Job drawing, mm, ordinate dimensions from the low corner. One solid piece. A direction names the side the tool comes from. Round coordinates to 2 decimals unless told otherwise and drop trailing zeros. Order: outer loops, then holes, each group sorted by start corner. A loop starts at its lowest first (then second) coordinate and runs counter-clockwise, first axis right, second up. Notation, with made-up numbers: (8, -21) -> (26, -21) arc R30 cw to (26, 5) -> close; hole circle Ø2 at (3.5, -5). An arc over 180 degrees is marked (long way). Write item = value, one per line.
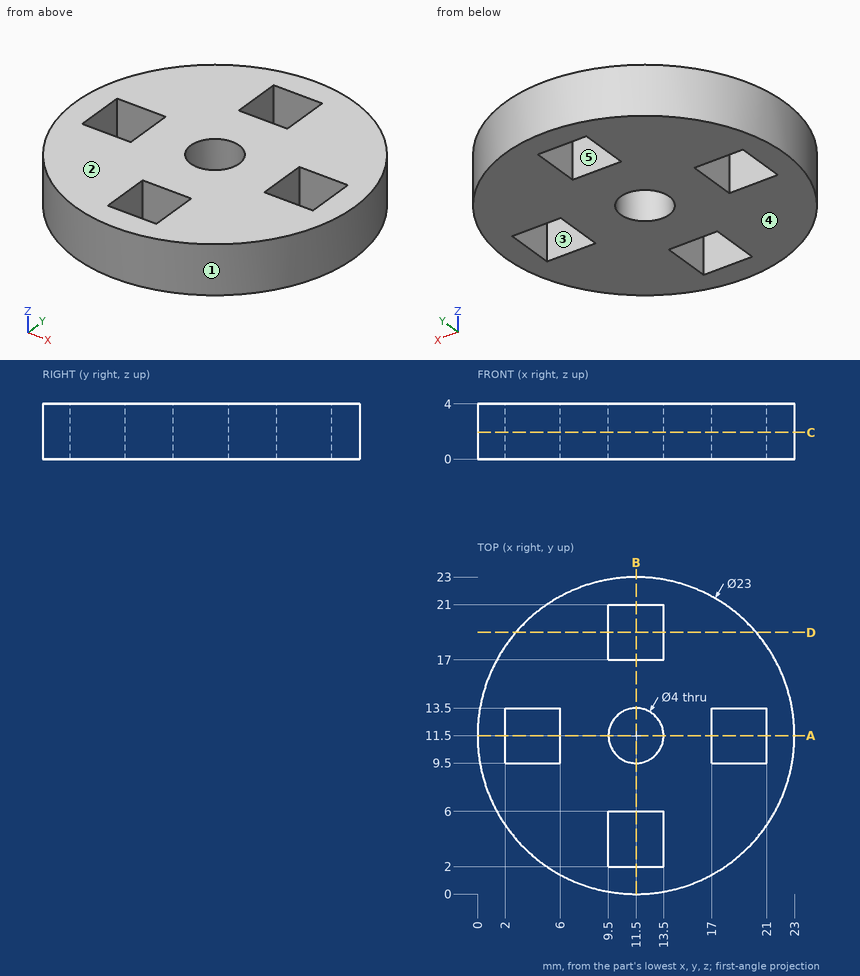
Q1. Probe probe 1 along Y at (x, z) = (11.5, 3.25); probe 2 along X at (y, z) = (10, 1.5); probe 3 along Y at (x, z) = (12, 1.65). List the from-to ranges inside material, lowest first.
Check values:
probe_1 = 0 to 2, 6 to 9.5, 13.5 to 17, 21 to 23
probe_2 = 0.1 to 2, 6 to 10.18, 12.82 to 17, 21 to 22.9
probe_3 = 0.01 to 2, 6 to 9.56, 13.44 to 17, 21 to 22.99
Q2. Cut at A-A, the plane y = 11.5. List the corners of the cut face in (x, z), and give its area (3 significant figures).
Check values:
outline = (0, 0) -> (2, 0) -> (2, 4) -> (0, 4) -> close; (6, 0) -> (9.5, 0) -> (9.5, 4) -> (6, 4) -> close; (13.5, 0) -> (17, 0) -> (17, 4) -> (13.5, 4) -> close; (21, 0) -> (23, 0) -> (23, 4) -> (21, 4) -> close
area = 44.0 mm²
Q3. Which spindle directions (+Z, -Z, +X, -X, +Y, -Y) get a long thin tool onto all of the face, cutting with end or side? Do the marked faces 4 and 5. Say none if no direction does.
Check values:
face_4 = -Z, +X, -X, +Y, -Y
face_5 = +Z, -Z
Q4. Flat gauge pins, fed straight in: pin 1 (1.2 mm diameter, centred on x = 4, z = 2, fed in from +Y); pin 2 (1.5 mm diameter, centred on x = 9.5, z = 3, fed in from +Y); pin 3 (2 mm diameter, centred on y = 4.5, z = 2, fed in from -X). Where does each tip first touch, or does it go through?
Check values:
pin_1 = 20.7
pin_2 = 22.93
pin_3 = 1.69
Q5. Mould opens along Y. For the marked faces 1, 2 and 3 say: released by +Y, released by -Y, zero draft, split by the parting line, or undercut.
Check values:
face_1 = split by the parting line
face_2 = zero draft
face_3 = undercut
Q6. Cut at C-C, the plane z = 1.95. List the corners of the cut face in (x, y), and give its area (3 significant figures).
Check values:
outline = circle Ø23 at (11.5, 11.5); hole (2, 9.5) -> (6, 9.5) -> (6, 13.5) -> (2, 13.5) -> close; hole (9.5, 2) -> (13.5, 2) -> (13.5, 6) -> (9.5, 6) -> close; hole circle Ø4 at (11.5, 11.5); hole (9.5, 17) -> (13.5, 17) -> (13.5, 21) -> (9.5, 21) -> close; hole (17, 9.5) -> (21, 9.5) -> (21, 13.5) -> (17, 13.5) -> close
area = 339 mm²
Q7. Cut at D-D, the plane y = 19. List the corners of the cut face in (x, z).
Check values:
outline = (2.78, 0) -> (9.5, 0) -> (9.5, 4) -> (2.78, 4) -> close; (13.5, 0) -> (20.22, 0) -> (20.22, 4) -> (13.5, 4) -> close
